from build123d import *

# Parameters (mm, degrees)
SKETCH1_W             = 60
SKETCH1_H             = 15
SKETCH1_R             = 3
BOSS_EXTRUDE1_DEPTH   = 6.35
M3_TAPPED_HOLE1_D     = 2.5
M3_TAPPED_HOLE1_DEPTH = 8.5
M3_TAPPED_HOLE1_TIP   = 0.751075774


with BuildPart() as part:
    # Sketch1 → Boss-Extrude1 (new body)
    with BuildSketch(Plane.XY):
        with Locations((30, 7.5)):
            Rectangle(SKETCH1_W, SKETCH1_H)
        with Locations((10, 7.5)):
            Circle(SKETCH1_R, mode=Mode.SUBTRACT)
        with Locations(Location((50, 7.5, 0), (0, 0, 180))):
            Circle(SKETCH1_R, mode=Mode.SUBTRACT)
    extrude(amount=BOSS_EXTRUDE1_DEPTH)

    # M3 Tapped Hole1
    with Locations(Plane(origin=(0, 15, 0), x_dir=(-1, 0, 0), z_dir=(0, 1, 0))):
        with Locations((-10, 3.175), (-50, 3.175)):
            Hole(M3_TAPPED_HOLE1_D / 2, depth=M3_TAPPED_HOLE1_DEPTH)
            with Locations((0, 0, -(M3_TAPPED_HOLE1_DEPTH + M3_TAPPED_HOLE1_TIP / 2))):  # 118° drill point
                Cone(0, M3_TAPPED_HOLE1_D / 2, M3_TAPPED_HOLE1_TIP, mode=Mode.SUBTRACT)


solid = part.part
Verification items for the finished model (mm, model axes). A direction names the side the tool comes from. Give positions to 0.01 mm unless a question says otherwise; leave off trailing zeros. Write each loop counter-clockwise with the first axis right and the second up, starting at its lowest first coordinate (ties: lowest second). Pieces come first, ordered by that corner, then holes.
(1) Cross-section at A-A (y = 7.5). Enter the section's corners in (x, z).
(2) Mould release check, pull along X, two halves, no side actions. Record for faces 1 (the face through (30, 8, 0)), 2 (the face through (51.192, 12.58, 3.55)), 3 (the face through (60, 7, 3)): +X half, -X half, draft (parallel to the pull), parting line (faces both ways), or undercut.
(3) Cross-section at C-C (z = 5). Enter the section's corners in (x, y), plus the area to 3 significant figures.
(4) Cross-section at D-D (x = 7.5). Enter the section's corners in (y, z).
(5) Material ranges on line 1 (Z direction, x = 50, y = 12.2) (3 decimals); line 2 (X direction, y = 9.5, z = 2.25); line 3 (Y direction, x = 10, z = 5.25), recorded low to high.
(6) Access from +Z, -Z, +X, -X, +Y, -Y to the whole of each face (thin tool, end or side, straight path). Record for faces 4 (the face through (11.384, 4.838, 3.131)), 5 (the face through (11.155, 12.58, 2.696)).
(7) Cross-section at B-B (x = 50). Enter the section's corners in (y, z) (3 decimals).
Worked out:
1. outline: (0, 0) - (7, 0) - (7, 6.35) - (0, 6.35) - close; (13, 0) - (47, 0) - (47, 6.35) - (13, 6.35) - close; (53, 0) - (60, 0) - (60, 6.35) - (53, 6.35) - close
2. face 1: draft
2. face 2: undercut
2. face 3: +X half
3. outline: (0, 0) - (60, 0) - (60, 15) - (0, 15) - close; hole circle Ø6 at (10, 7.5); hole circle Ø6 at (50, 7.5)
3. area: 843 mm2
4. outline: (0, 0) - (5.84, 0) - (5.84, 6.35) - (0, 6.35) - close; (9.16, 0) - (15, 0) - (15, 6.35) - (9.16, 6.35) - close
5. line 1: z = 0 to 1.925, 4.425 to 6.35
5. line 2: x = 0 to 7.76, 12.24 to 47.76, 52.24 to 60
5. line 3: y = 0 to 4.5, 10.5 to 15
6. face 4: +Z, -Z
6. face 5: +Y
7. outline: (0, 0) - (4.5, 0) - (4.5, 6.35) - (0, 6.35) - close; (10.5, 0) - (15, 0) - (15, 1.925) - (10.5, 1.925) - close; (10.5, 4.425) - (15, 4.425) - (15, 6.35) - (10.5, 6.35) - close
